Verification items for this drawing (mm, ordinates from the low corner). A direction names the side the tool comes from. Round coordinates to 2 decimals unless told otherwise and drop trailing zeros. Loops run counter-clockwise (first coordinate to the right, second up) from the corner with the lowest first, then second, coordinate; pieces in that order, holes last. Notation, with made-up numbers: M 37.5,78 L 73.5,78 A27 ccw 73.5,102 Z; hole C -30.75,37 d11. An arc over 180 degrees is marked long. One line per item, written item: value.
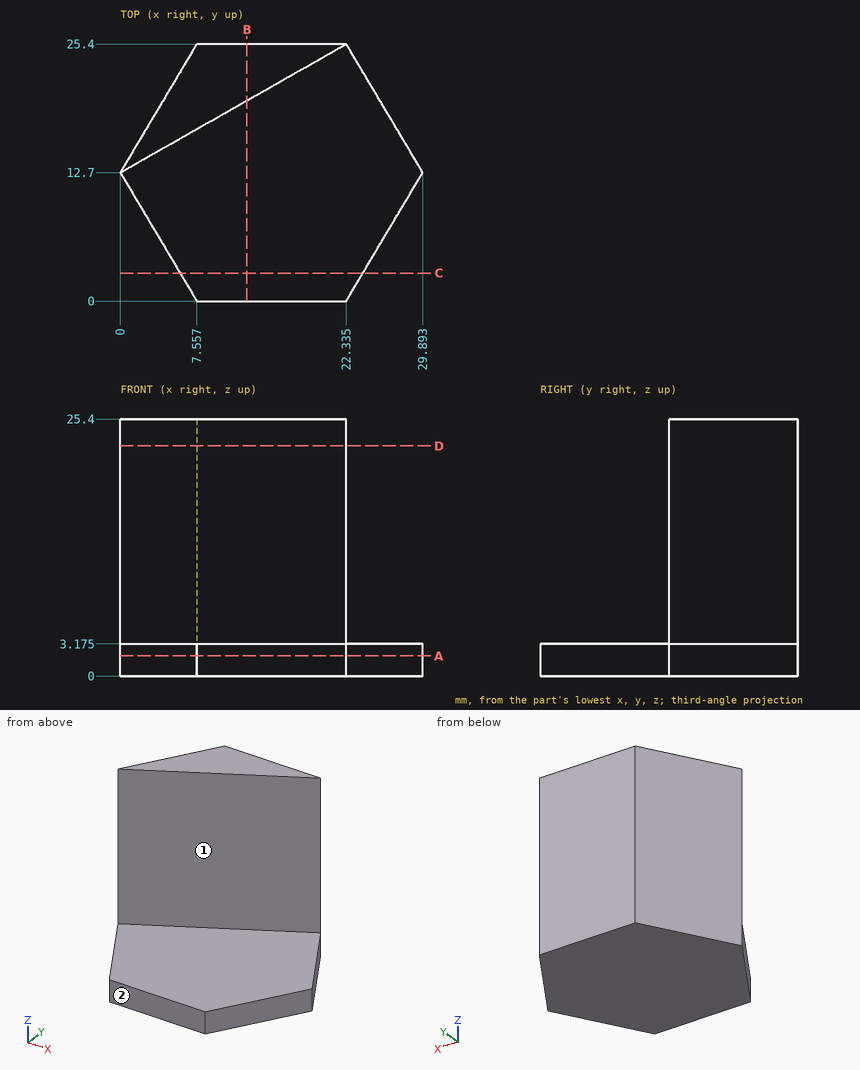
(1) Tool access check on the marked faces 1 and 2. Record the directions out of +Z, -Z, +X, -X, +Y, -Y that give a thin tool (end or side, any length) a straight path to the whole face; none if there is none.
Completed:
face 1: +Z, +X, -Y
face 2: +Z, -Z, +X, -X, -Y
(2) Thickness scan on L1, parallel to Z at x = 23.5, y = 12.75 (1 decimal); L2, parallel to Y at x = 12.75, z = 12.25; L3, parallel to Y at x = 10.75, z = 18. Record the ranges inside material, lowest first. Write a range as from..to.
Completed:
L1: z = 0..3.2
L2: y = 19.95..25.4
L3: y = 18.81..25.4
(3) Sectioned sample at D-D on z = 22.75. Enter the section's corners in (x, y) (1 decimal).
Completed:
outline: M 0,12.7 L 22.3,25.4 L 7.6,25.4 Z
(4) Depth check by flat-ended pin: pin 1 Ø2 at (y, z) = (14.5, 22.5) entering from -X (1 decimal); pin 2 Ø8 at (y, z) = (21.5, 21.5) entering from +X (1 decimal); pin 3 Ø1 at (x, y) = (23.5, 3.5) entering from +Z (3 decimals); pin 4 Ø3 at (y, z) = (9.5, 10.5) entering from -X (3 decimals). Enter the tip coordinate at first touch or a pass-through.
Completed:
pin 1: stops at x = 0.5
pin 2: stops at x = 22.3
pin 3: stops at z = 3.175
pin 4: passes through
(5) Sectioned sample at A-A on z = 2. Enter the section's corners in (x, y) (1 decimal), and give its area (3 significant figures).
Completed:
outline: M 0,12.7 L 7.6,0 L 22.3,0 L 29.9,12.7 L 22.3,25.4 L 7.6,25.4 Z
area: 567 mm^2
(6) Sectioned sample at B-B on x = 12.5. Enter the section's corners in (y, z) (1 decimal), and give its area (3 significant figures).
Completed:
outline: M 0,0 L 25.4,0 L 25.4,25.4 L 19.8,25.4 L 19.8,3.2 L 0,3.2 Z
area: 205 mm^2
(7) Sectioned sample at C-C on y = 2.75. Enter the section's corners in (x, z) (1 decimal).
Completed:
outline: M 5.9,0 L 24,0 L 24,3.2 L 5.9,3.2 Z
